For this review, take the finished solid that the model builds, in its own axes (mm). Face numbers are marked on the shaded views. A direction names the side the tool comes from. Coordinates: 2 decimals unless noted, no trailing zeros. Loops run counter-clockwise (first coordinate to the right, second up) from the corner with the lowest first, then second, coordinate; pieces in that order, holes last. Notation, with made-up numbers: M -36.75,23.25 L -32.75,23.25 A16 ccw -32.75,35.25 Z; hole C -18.5,-26.5 d8. An arc over 180 degrees is marked long. Write item = value, one per line.
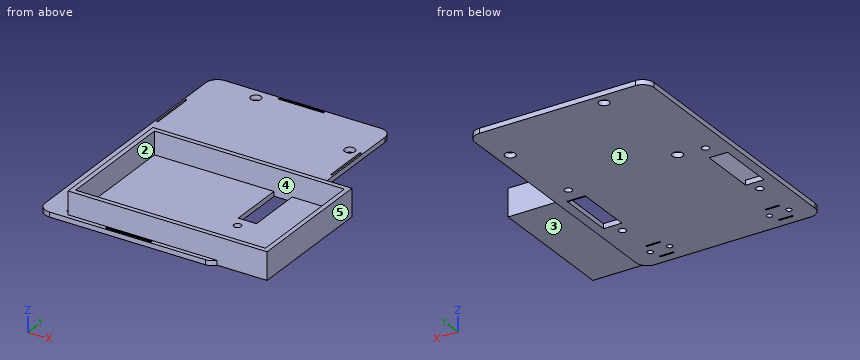
from build123d import *

# Parameters (mm, degrees)
SKETCH1_W                    = 78.2
SKETCH1_H                    = 120
SKETCH1_R                    = 2.25
BOSS_EXTRUDE1_DEPTH          = 2.1
CUT_EXTRUDE1_REACH           = 4.1
SKETCH2_R                    = 1.2
SKETCH2_W                    = 6.1
SKETCH2_H                    = 0.6
CUT_EXTRUDE3_REACH           = 4.1
SKETCH8_R                    = 1.6
SKETCH8_W                    = 8
SKETCH8_H                    = 25
FILLET2_R                    = 5
SCHIZZO2_W                   = 87
SCHIZZO2_H                   = 58
SCHIZZO2_W_2                 = 83
SCHIZZO2_H_2                 = 54
ESTRUSIONE_ESTRUSIONE1_DEPTH = 10
SCHIZZO3_W                   = 0.7
SCHIZZO3_H                   = 20
SCHIZZO3_W_2                 = 20
SCHIZZO3_H_2                 = 0.7
SCHIZZO3_H_3                 = 0.65
TAGLIO_ESTRUSIONE1_DEPTH     = 1
SCHIZZO2_3_W                 = 8
SCHIZZO2_3_H                 = 0.6
SCHIZZO2_3_W_2               = 2
ESTRUSIONE_ESTRUSIONE2_DEPTH = 2


with BuildPart() as part:
    # Sketch1 → Boss-Extrude1 (new body)
    with BuildSketch(Plane.XY):
        Rectangle(SKETCH1_W, SKETCH1_H)
        with Locations((-17.3, 55)):
            Circle(SKETCH1_R, mode=Mode.SUBTRACT)
        with Locations((33.5, 39.76)):
            Circle(SKETCH1_R, mode=Mode.SUBTRACT)
        with Locations((-18.6, 6.74)):
            Circle(SKETCH1_R, mode=Mode.SUBTRACT)
    extrude(amount=BOSS_EXTRUDE1_DEPTH)

    # Sketch2 → Cut-Extrude1 (cut, up to next)
    with BuildSketch(Plane.XY.offset(2.1), mode=Mode.PRIVATE) as cut_extrude1_sk1:
        with Locations((-30.3, -51)):
            Circle(SKETCH2_R)
    cut_extrude1_tool1 = extrude(cut_extrude1_sk1.sketch, amount=-CUT_EXTRUDE1_REACH, mode=Mode.PRIVATE) & part.part
    add(cut_extrude1_tool1.solids().sort_by_distance((-30.3, -51, 2.1))[0], mode=Mode.SUBTRACT)
    # Sketch2 → Cut-Extrude1 (cut, up to next)
    with BuildSketch(Plane.XY.offset(2.1), mode=Mode.PRIVATE) as cut_extrude1_sk2:
        with Locations((-21.8, -51)):
            Circle(SKETCH2_R)
    cut_extrude1_tool2 = extrude(cut_extrude1_sk2.sketch, amount=-CUT_EXTRUDE1_REACH, mode=Mode.PRIVATE) & part.part
    add(cut_extrude1_tool2.solids().sort_by_distance((-21.8, -51, 2.1))[0], mode=Mode.SUBTRACT)
    # Sketch2 → Cut-Extrude1 (cut, up to next)
    with BuildSketch(Plane.XY.offset(2.1), mode=Mode.PRIVATE) as cut_extrude1_sk3:
        with Locations((21.8, -51)):
            Circle(SKETCH2_R)
    cut_extrude1_tool3 = extrude(cut_extrude1_sk3.sketch, amount=-CUT_EXTRUDE1_REACH, mode=Mode.PRIVATE) & part.part
    add(cut_extrude1_tool3.solids().sort_by_distance((21.8, -51, 2.1))[0], mode=Mode.SUBTRACT)
    # Sketch2 → Cut-Extrude1 (cut, up to next)
    with BuildSketch(Plane.XY.offset(2.1), mode=Mode.PRIVATE) as cut_extrude1_sk4:
        with Locations((30.3, -51)):
            Circle(SKETCH2_R)
    cut_extrude1_tool4 = extrude(cut_extrude1_sk4.sketch, amount=-CUT_EXTRUDE1_REACH, mode=Mode.PRIVATE) & part.part
    add(cut_extrude1_tool4.solids().sort_by_distance((30.3, -51, 2.1))[0], mode=Mode.SUBTRACT)
    # Sketch2 → Cut-Extrude1 (cut, up to next)
    with BuildSketch(Plane.XY.offset(2.1), mode=Mode.PRIVATE) as cut_extrude1_sk5:
        with Locations((-26.05, -46.3)):
            Rectangle(SKETCH2_W, SKETCH2_H)
    cut_extrude1_tool5 = extrude(cut_extrude1_sk5.sketch, amount=-CUT_EXTRUDE1_REACH, mode=Mode.PRIVATE) & part.part
    add(cut_extrude1_tool5.solids().sort_by_distance((-26.05, -46.3, 2.1))[0], mode=Mode.SUBTRACT)
    # Sketch2 → Cut-Extrude1 (cut, up to next)
    with BuildSketch(Plane.XY.offset(2.1), mode=Mode.PRIVATE) as cut_extrude1_sk6:
        with Locations((-26.05, -55.7)):
            Rectangle(SKETCH2_W, SKETCH2_H)
    cut_extrude1_tool6 = extrude(cut_extrude1_sk6.sketch, amount=-CUT_EXTRUDE1_REACH, mode=Mode.PRIVATE) & part.part
    add(cut_extrude1_tool6.solids().sort_by_distance((-26.05, -55.7, 2.1))[0], mode=Mode.SUBTRACT)
    # Sketch2 → Cut-Extrude1 (cut, up to next)
    with BuildSketch(Plane.XY.offset(2.1), mode=Mode.PRIVATE) as cut_extrude1_sk7:
        with Locations((26.05, -55.7)):
            Rectangle(SKETCH2_W, SKETCH2_H)
    cut_extrude1_tool7 = extrude(cut_extrude1_sk7.sketch, amount=-CUT_EXTRUDE1_REACH, mode=Mode.PRIVATE) & part.part
    add(cut_extrude1_tool7.solids().sort_by_distance((26.05, -55.7, 2.1))[0], mode=Mode.SUBTRACT)
    # Sketch2 → Cut-Extrude1 (cut, up to next)
    with BuildSketch(Plane.XY.offset(2.1), mode=Mode.PRIVATE) as cut_extrude1_sk8:
        with Locations((26.05, -46.3)):
            Rectangle(SKETCH2_W, SKETCH2_H)
    cut_extrude1_tool8 = extrude(cut_extrude1_sk8.sketch, amount=-CUT_EXTRUDE1_REACH, mode=Mode.PRIVATE) & part.part
    add(cut_extrude1_tool8.solids().sort_by_distance((26.05, -46.3, 2.1))[0], mode=Mode.SUBTRACT)

    # Sketch8 → Cut-Extrude3 (cut, up to next)
    with BuildSketch(Plane.XY.offset(2.1), mode=Mode.PRIVATE) as cut_extrude3_sk1:
        with Locations((-30, -31.5)):
            Circle(SKETCH8_R)
    cut_extrude3_tool1 = extrude(cut_extrude3_sk1.sketch, amount=-CUT_EXTRUDE3_REACH, mode=Mode.PRIVATE) & part.part
    add(cut_extrude3_tool1.solids().sort_by_distance((-30, -31.5, 2.1))[0], mode=Mode.SUBTRACT)
    # Sketch8 → Cut-Extrude3 (cut, up to next)
    with BuildSketch(Plane.XY.offset(2.1), mode=Mode.PRIVATE) as cut_extrude3_sk2:
        with Locations((30, -31.5)):
            Circle(SKETCH8_R)
    cut_extrude3_tool2 = extrude(cut_extrude3_sk2.sketch, amount=-CUT_EXTRUDE3_REACH, mode=Mode.PRIVATE) & part.part
    add(cut_extrude3_tool2.solids().sort_by_distance((30, -31.5, 2.1))[0], mode=Mode.SUBTRACT)
    # Sketch8 → Cut-Extrude3 (cut, up to next)
    with BuildSketch(Plane.XY.offset(2.1), mode=Mode.PRIVATE) as cut_extrude3_sk3:
        with Locations((30, 5.5)):
            Circle(SKETCH8_R)
    cut_extrude3_tool3 = extrude(cut_extrude3_sk3.sketch, amount=-CUT_EXTRUDE3_REACH, mode=Mode.PRIVATE) & part.part
    add(cut_extrude3_tool3.solids().sort_by_distance((30, 5.5, 2.1))[0], mode=Mode.SUBTRACT)
    # Sketch8 → Cut-Extrude3 (cut, up to next)
    with BuildSketch(Plane.XY.offset(2.1), mode=Mode.PRIVATE) as cut_extrude3_sk4:
        with Locations((-30, 5.5)):
            Circle(SKETCH8_R)
    cut_extrude3_tool4 = extrude(cut_extrude3_sk4.sketch, amount=-CUT_EXTRUDE3_REACH, mode=Mode.PRIVATE) & part.part
    add(cut_extrude3_tool4.solids().sort_by_distance((-30, 5.5, 2.1))[0], mode=Mode.SUBTRACT)
    # Sketch8 → Cut-Extrude3 (cut, up to next)
    with BuildSketch(Plane.XY.offset(2.1), mode=Mode.PRIVATE) as cut_extrude3_sk5:
        with Locations((-31.1, -14)):
            Rectangle(SKETCH8_W, SKETCH8_H)
    cut_extrude3_tool5 = extrude(cut_extrude3_sk5.sketch, amount=-CUT_EXTRUDE3_REACH, mode=Mode.PRIVATE) & part.part
    add(cut_extrude3_tool5.solids().sort_by_distance((-31.1, -14, 2.1))[0], mode=Mode.SUBTRACT)
    # Sketch8 → Cut-Extrude3 (cut, up to next)
    with BuildSketch(Plane.XY.offset(2.1), mode=Mode.PRIVATE) as cut_extrude3_sk6:
        with Locations((31.1, -14)):
            Rectangle(SKETCH8_W, SKETCH8_H)
    cut_extrude3_tool6 = extrude(cut_extrude3_sk6.sketch, amount=-CUT_EXTRUDE3_REACH, mode=Mode.PRIVATE) & part.part
    add(cut_extrude3_tool6.solids().sort_by_distance((31.1, -14, 2.1))[0], mode=Mode.SUBTRACT)

    # Fillet2
    fillet2_edges = [part.edges().sort_by_distance(p)[0] for p in [
        (39.1, -60, 1.05),
        (-39.1, -60, 1.05),
        (-39.1, 60, 1.05),
        (39.1, 60, 1.05),
    ]]
    fillet(fillet2_edges, radius=FILLET2_R)

    # Schizzo2 → Estrusione-Estrusione1 (add)
    with BuildSketch(Plane.XY.offset(2.1)):
        with Locations((16.4, -29.1)):
            Rectangle(SCHIZZO2_W, SCHIZZO2_H)
        with Locations((16.4, -29.1)):
            Rectangle(SCHIZZO2_W_2, SCHIZZO2_H_2, mode=Mode.SUBTRACT)
    extrude(amount=ESTRUSIONE_ESTRUSIONE1_DEPTH)

    # Schizzo3 → Taglio-Estrusione1 (cut)
    with BuildSketch(Plane.XY.offset(2.1)):
        with Locations((-38.1, 30)):
            Rectangle(SCHIZZO3_W, SCHIZZO3_H)
        with Locations((38.1, 30)):
            Rectangle(SCHIZZO3_W, SCHIZZO3_H)
        with Locations((0, 59)):
            Rectangle(SCHIZZO3_W_2, SCHIZZO3_H_2)
        with Locations((0, -58.975)):
            Rectangle(SCHIZZO3_W_2, SCHIZZO3_H_3)
    extrude(amount=-TAGLIO_ESTRUSIONE1_DEPTH, mode=Mode.SUBTRACT)

    # Schizzo2<3> → Estrusione-Estrusione2 (add)
    with BuildSketch(Plane.XY.offset(2.1)):
        with Locations((31.1, -1.8)):
            Rectangle(SCHIZZO2_3_W, SCHIZZO2_3_H)
        with Locations((-26.1, -46.3)):
            Rectangle(SCHIZZO2_3_W_2, SCHIZZO2_3_H)
        with BuildLine():
            Line((39.1, -0.1), (39.1, -55))
            ThreePointArc((39.1, -55), (38.823084016, -56.640877015), (38.023009049, -58.1))
            Line((38.023009049, -58.1), (59.9, -58.1))
            Line((59.9, -58.1), (59.9, -0.1))
            Line((59.9, -0.1), (39.1, -0.1))
        make_face()
        with Locations((-26.1, -55.7)):
            Rectangle(SCHIZZO2_3_W_2, SCHIZZO2_3_H)
    extrude(amount=-ESTRUSIONE_ESTRUSIONE2_DEPTH)


solid = part.part
Q1. Machinability: for the marked faces 1 and 2, which of the approach directions +Z, -Z, +X, -X, +Y, -Y give a long, thin tool a straight path to every point of the face, cutting with its end or side? Answer none if there is none.
Solved:
face_1 = -Z, +X, -X, +Y, -Y
face_2 = +Z
Q2. For pin 1 Ø1 at (y, z) = (6, 1.5) entering from +X; pin 2 Ø0.5 at (y, z) = (-59, 1.5) entering from -X; pin 3 Ø1.5 at (x, z) = (0.5, 3.5) entering from -Y, all flat-tipped, find the tip position at first contact; note any pin that passes through.
Solved:
pin_1 = 39.1
pin_2 = -37.41
pin_3 = -58.1
Q3. Add section A-A (y = -17.5). Write out the cut boundary in (x, z), and give its area (3 significant figures).
Solved:
outline = M -39.1,0 L -35.1,0 L -35.1,2.1 L -39.1,2.1 Z; M -27.1,0 L 27.1,0 L 27.1,2.1 L -25.1,2.1 L -25.1,12.1 L -27.1,12.1 Z; M 35.1,0 L 39.1,0 L 39.1,0.1 L 59.9,0.1 L 59.9,12.1 L 57.9,12.1 L 57.9,2.1 L 35.1,2.1 Z
area = 212 mm²
Q4. For line 1 along Y through (x, z) = (18, 4.5); line 2 along X through (y, z) = (-4.5, 9); line 3 along Y through (x, z) = (-24, 2), list the stretches that pass through material, from the lowest coordinate up.
Solved:
line_1 = -58.1 to -56.1, -2.1 to -0.1
line_2 = -27.1 to -25.1, 57.9 to 59.9
line_3 = -60 to -56, -55.4 to -46.6, -46 to 60
Q5. Add section C-C (x = 50). Write out the cut boundary in (y, z), and give its area (3 significant figures).
Solved:
outline = M -58.1,0.1 L -0.1,0.1 L -0.1,12.1 L -2.1,12.1 L -2.1,2.1 L -56.1,2.1 L -56.1,12.1 L -58.1,12.1 Z
area = 156 mm²
Q6. Draft analysis for pull direction X (two halves, no side actions). For the marked faces 3, 4 and 5, state which applies: +X half, -X half, draft (parallel to the pull), parting line (faces both ways), or undercut.
Solved:
face_3 = draft
face_4 = undercut
face_5 = +X half
Q7. Add section B-B (z = 4.75). Write out the cut boundary in (x, y), and give its area (3 significant figures).
Solved:
outline = M -27.1,-58.1 L 59.9,-58.1 L 59.9,-0.1 L -27.1,-0.1 Z; hole M -25.1,-56.1 L 57.9,-56.1 L 57.9,-2.1 L -25.1,-2.1 Z
area = 564 mm²
Q8. Add section D-D (y = 24.5). Write out the cut boundary in (x, z).
Solved:
outline = M -39.1,0 L 39.1,0 L 39.1,2.1 L 38.45,2.1 L 38.45,1.1 L 37.75,1.1 L 37.75,2.1 L -37.75,2.1 L -37.75,1.1 L -38.45,1.1 L -38.45,2.1 L -39.1,2.1 Z
